The model under review builds one solid part; all positions refer to its coordinate system, in mm. Face numbers are marked on the shaded views. Round coordinates to 2 decimals unless told otherwise and drop trailing zeros. Loops run counter-clockwise (first coordinate to the right, second up) from the corner with the lowest first, then second, coordinate; pieces in that order, holes last. Notation, with made-up numbers: (-37, -25.5) -> (-10, -25.5) arc R23 cw to (-10, 12.5) -> close; hole circle Ø9 at (16, 50.25). An arc over 180 degrees is marked (long way). Return JSON: item names as keys, results as strings. Group by question number.
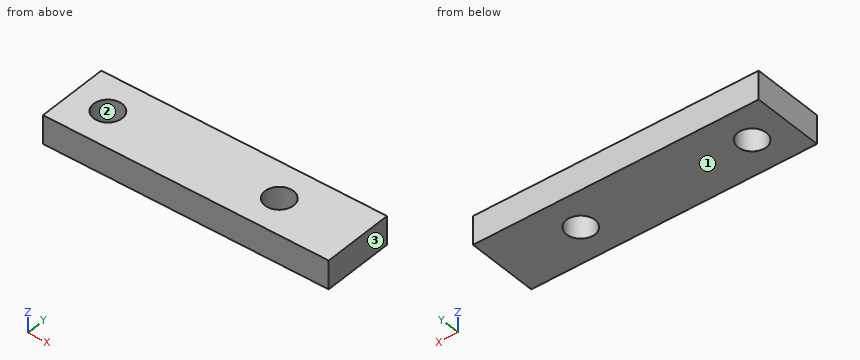
Autodesk Inventor part; units mm, degrees
ref_plane "YZ Plane" through (0, 0, 0) normal (1, 0, 0) x (0, 1, 0)
ref_plane "XZ Plane" through (0, 0, 0) normal (0, 1, 0) x (-1, 0, 0)
ref_plane "XY Plane" through (0, 0, 0) normal (0, 0, 1) x (1, 0, 0)
sketch "Sketch1" plane through (0, 0, 0) normal (0, 0, 1) x (1, 0, 0)
  circle A0 centre (0, 0) radius 4
  line L0 (0, 0) -> (48, 0)
  circle A1 centre (48, 0) radius 4
  line L1 (0, 0) -> (0, 10)
  line L2 (0, 10) -> (70, 10)
  line L3 (70, 10) -> (70, -10)
  line L4 (70, -10) -> (-10, -10)
  line L5 (-10, -10) -> (-10, 10)
  line L6 (-10, 10) -> (0, 10)
  dimension "d0" = 8
  dimension "d1" = 48
  dimension "d2" = 8
  dimension "d3" = 10
  dimension "d4" = 70
  dimension "d5" = 20
  dimension "d6" = 80
extrude "Extrusion1" add sketch "Sketch1" along normal blind 8
properties part number "plaque 1"
1. Draft analysis for pull direction X (two halves, no side actions). For the marked faces 1, 2 and 3, state which applies: pulls with the +X half, pulls with the -X half, needs draft (parallel to the pull), parting line crosses it, or undercut.
2. Wall thickness on line 1 (X direction, y = 0, z = 4.5); line 2 (Y direction, x = 48, z = 6.5); line 3 (X direction, y = -3, z = 6.5): over which ranges is each line inside the solid? List them lowest first.
3. We need section B-B, the plane x = 0. Write out the cut boundary in (y, z), then the cut area to 3 significant figures.
4. We need section A-A, the plane y = 0. Write out the cut boundary in (x, z).
5. For P1, Ø5, axis at x = 48, y = 0, coming from the -Z side, flat-tipped, find the tip position at first contact; note if it passes through.
6. We need section C-C, the plane z = 6.25. Write out the cut boundary in (x, y).
7. We need section D-D, the plane x = 46.5. Write out the cut boundary in (y, z), then the cut area to 3 significant figures.
Check sheet entries:
{
 "1": {"face 1": "needs draft", "face 2": "undercut", "face 3": "pulls with the +X half"},
 "2": {"line 1": "x = -10 to -4, 4 to 44, 52 to 70", "line 2": "y = -10 to -4, 4 to 10", "line 3": "x = -10 to -2.65, 2.65 to 45.35, 50.65 to 70"},
 "3": {"outline": "(-10, 0) -> (-4, 0) -> (-4, 8) -> (-10, 8) -> close; (4, 0) -> (10, 0) -> (10, 8) -> (4, 8) -> close", "area": "96.0 mm²"},
 "4": {"outline": "(-10, 0) -> (-4, 0) -> (-4, 8) -> (-10, 8) -> close; (4, 0) -> (44, 0) -> (44, 8) -> (4, 8) -> close; (52, 0) -> (70, 0) -> (70, 8) -> (52, 8) -> close"},
 "5": {"P1": "passes through"},
 "6": {"outline": "(-10, -10) -> (70, -10) -> (70, 10) -> (-10, 10) -> close; hole circle Ø8 at (0, 0); hole circle Ø8 at (48, 0)"},
 "7": {"outline": "(-10, 0) -> (-3.71, 0) -> (-3.71, 8) -> (-10, 8) -> close; (3.71, 0) -> (10, 0) -> (10, 8) -> (3.71, 8) -> close", "area": "101 mm²"}
}
